from build123d import *

# Parameters (mm, degrees)
ESQUISSE1_R             = 7.366
BOSS_EXTRU_1_DEPTH      = 9.398
BOSS_EXTRU_2_START      = -2.1844
BOSS_EXTRU_2_DEPTH      = 2.1844
CONG_1_R                = 2.54
ESQUISSE3_R             = 1.143
ENL_V_MAT_EXTRU_2_DEPTH = 16.678200152


with BuildPart() as part:
    # Esquisse1 → Boss.-Extru.1 (new body)
    with BuildSketch(Plane.XY):
        Circle(ESQUISSE1_R)
    extrude(amount=BOSS_EXTRU_1_DEPTH)

    # Esquisse2 → Boss.-Extru.2 (add)
    with BuildSketch(Plane.XY.offset(9.398).offset(BOSS_EXTRU_2_START)):
        with BuildLine():
            Line((7.366, 2.794), (6.815535195, 2.794))
            ThreePointArc((6.815535195, 2.794), (7.22707369, 1.423854584), (7.366, 0))
            Line((7.366, 0), (10.16, 0))
            ThreePointArc((10.16, 0), (9.341656347, 1.975656347), (7.366, 2.794))
        make_face()
        with BuildLine():
            Line((10.16, 0), (7.366, 0))
            ThreePointArc((7.366, 0), (7.22707369, -1.423854584), (6.815535195, -2.794))
            Line((6.815535195, -2.794), (7.366, -2.794))
            ThreePointArc((7.366, -2.794), (9.341656347, -1.975656347), (10.16, 0))
        make_face()
        with BuildLine():
            Line((-7.366, 0), (-10.16, 0))
            ThreePointArc((-10.16, 0), (-9.341656347, -1.975656347), (-7.366, -2.794))
            Line((-7.366, -2.794), (-6.815535195, -2.794))
            ThreePointArc((-6.815535195, -2.794), (-7.22707369, -1.423854584), (-7.366, 0))
        make_face()
        with BuildLine():
            Line((-6.815535195, 2.794), (-7.366, 2.794))
            ThreePointArc((-7.366, 2.794), (-9.341656347, 1.975656347), (-10.16, 0))
            Line((-10.16, 0), (-7.366, 0))
            ThreePointArc((-7.366, 0), (-7.22707369, 1.423854584), (-6.815535195, 2.794))
        make_face()
    extrude(amount=BOSS_EXTRU_2_DEPTH)

    # Congé1
    # the kernel refuses this fillet: 2.54 mm, written as the material it adds along each edge
    with BuildSketch(Plane(origin=(6.815535195, 2.794, 7.2136), x_dir=(-0.45524151464262924, 0.8903679932173465, 0), z_dir=(0, 0, 1)), Plane(origin=(-6.815535195, -2.794, 7.2136), x_dir=(0.4552415146426176, -0.8903679932173524, 0), z_dir=(0, 0, 1))) as cong_1_piece_1:
        with BuildLine():
            CenterArc((1.442130851, -2.531130754), CONG_1_R, 94.789504406, 46.813825589)
            Line((-0.548542223, -0.953531086), (-0.74760953, -0.795771119))
            ThreePointArc((-0.74760953, -0.795771119), (-0.476747902, -0.374484899), (-0.22615347, 0.115631345))
            Line((-0.22615347, 0.115631345), (0.021207807, 0.253113075))
            ThreePointArc((0.021207807, 0.253113075), (0.615026392, 0.228279187), (1.208844978, 0.253113075))
            Line((1.208844978, 0.253113075), (1.230052785, 0))
        make_face()
    extrude(amount=2.1844)
    with BuildSketch(Plane(origin=(6.815535195, -2.794, 7.2136), x_dir=(-0.4552415146426287, -0.8903679932173468, 0), z_dir=(0, 0, 1)), Plane(origin=(-6.815535195, 2.794, 7.2136), x_dir=(0.45524151464261825, 0.890367993217352, 0), z_dir=(0, 0, 1))) as cong_1_piece_2:
        with BuildLine():
            CenterArc((1.442130851, 2.531130754), CONG_1_R, 218.396670004, 46.813825589)
            Line((-0.548542223, 0.953531086), (-0.74760953, 0.795771119))
            ThreePointArc((-0.74760953, 0.795771119), (-0.476747902, 0.374484899), (-0.22615347, -0.115631345))
            Line((-0.22615347, -0.115631345), (0.021207807, -0.253113075))
            ThreePointArc((0.021207807, -0.253113075), (0.615026392, -0.228279187), (1.208844978, -0.253113075))
            Line((1.208844978, -0.253113075), (1.230052785, 0))
        make_face()
    extrude(amount=2.1844)

    # Esquisse3 → Enlèv. mat.-Extru.2 (cut, through all)
    with BuildSketch(Plane.XY.offset(9.398)):
        with Locations((-7.366, 0)):
            Circle(ESQUISSE3_R)
        with Locations((7.366, 0)):
            Circle(ESQUISSE3_R)
    extrude(amount=-ENL_V_MAT_EXTRU_2_DEPTH, mode=Mode.SUBTRACT)

    # Esquisse4 → Révolution4 (revolve)
    with BuildSketch(Plane(origin=(0, 0, 0), x_dir=(0, 0, -1), z_dir=(1, 0, 0))):
        with BuildLine():
            Line((-8.4836, 0), (4.064, 0))
            ThreePointArc((4.064, 0), (-2.2098, 6.2738), (-8.4836, 0))
        make_face()
    revolve(axis=Axis((0, 0, 7.037287666), (0, 0, -1)))


solid = part.part
Work out the finished part from the listing and answer in its coordinate system (mm). A direction names the side the tool comes from. Give positions to 0.01 mm unless a question says otherwise; leave off trailing zeros. Write each loop counter-clockwise with the first axis right and the second up, starting at its lowest first coordinate (ties: lowest second). Pieces come first, ordered by that corner, then holes. Notation, with made-up numbers: (23.25, -26.5) - (50.25, -26.5) arc R19 cw to (50.25, -8.5) - close; hole circle Ø3 at (-23.5, 87.5). An arc over 180 degrees is marked (long way). One line per item, written item: value. Start each with the question number.
1. For faces 5 (the flat face through (1, 6, 0)), 6 (the cylindrical face through (-0.146, -7.365, 4.633)), 7 (the cylindrical face through (0.146, 7.365, 4.633)), 8 (the cylindrical face through (6.954, 3.151, 8.291)), determine the directions among +Z, -Z, +X, -X, +Y, -Y from which every point of the face is accessible in a straight line to the end or side of a thin tool.
2. Given pin 1 (6 mm diameter, centred on y = 1, z = 1, fed in from +X); pin 2 (6 mm diameter, centred on y = -1.5, z = 2, fed in from -X); pin 3 (2 mm diameter, centred on x = 2, y = -4.5, fed in from -Z); pin 4 (1.8 mm diameter, centred on x = -7.366, y = 0, fed in from +Z) (3 decimals), each flat-ended and moving along its own axis, determine where each tip first touches the part or whether it passes through.
3. Consider probe 1 along X at (y, z) = (-0.25, 7.5); probe 2 along Z at (x, y) = (2.5, 6.5); probe 3 along Y at (x, z) = (-6.75, 6). Determine where each line is inside the solid, lowest interval first.
4. For a pull along X with two mould halves and no side action, classify faces 1 (the cylindrical face through (-6.31, -0.44, 5.81)), 2 (the cylindrical face through (-6.978, 3.134, 8.291)), 3 (the cylindrical face through (6.978, -3.134, 8.291)), 4 (the cylindrical face through (6.224, 0.05, 5.809)) as +X half, -X half, draft (parallel to the pull), parting line (faces both ways), or undercut.
5. Find section B-B (y = 3.5). Write down the section's boundary in (x, z), then the cut area to 3 significant figures.
6. Find section A-A (z = 5). Write down the section's boundary in (x, y).
7. Find section C-C (x = 2.75). Write down the section's boundary in (y, z), then the cut area to 3 significant figures.
8. Find section D-D (y = -2.5). Write down the section's boundary in (x, z), then the cut area to 3 significant figures.
Geometry results:
1. face 5: -Z
1. face 6: -Z, -Y
1. face 7: -Z, +Y
1. face 8: +Z, -Z, +X, +Y
2. pin 1: x = 7.28
2. pin 2: x = -7.28
2. pin 3: z = -2.69
2. pin 4: through
3. probe 1: -10.15 to -8.48, -6.25 to 6.25, 8.48 to 10.15
3. probe 2: 0 to 9.4
3. probe 3: -2.95 to -0.96, 0.96 to 2.95
4. face 1: undercut
4. face 2: -X half
4. face 3: +X half
4. face 4: undercut
5. outline: (-6.55, 7.21) - (-6.48, 7.21) - (-6.48, 0) - (-4.71, 0) arc R5.21 ccw to (4.71, 0) - (6.48, 0) - (6.48, 7.21) - (6.55, 7.21) - (6.55, 9.4) - (-6.55, 9.4) - close
5. area: 142 mm2
6. outline: (-7.28, -1.14) arc R7.37 ccw to (7.28, -1.14) arc R1.14 cw to (7.28, 1.14) arc R7.37 ccw to (-7.28, 1.14) arc R1.14 cw to start
7. outline: (-6.83, 0) - (-5.19, 0) arc R5.64 ccw to (5.19, 0) - (6.83, 0) - (6.83, 9.4) - (-6.83, 9.4) - close
7. area: 154 mm2
8. outline: (-8.61, 7.21) - (-6.93, 7.21) - (-6.93, 0) - (-5.31, 0) arc R5.75 ccw to (5.31, 0) - (6.93, 0) - (6.93, 7.21) - (8.61, 7.21) - (8.61, 9.4) - (-8.61, 9.4) - close
8. area: 165 mm2
